```python
from build123d import *

# Parameters (mm, degrees)
ESQUISSE3_R             = 1.5
ESQUISSE3_R_2           = 2
ENL_V_MAT_EXTRU_2_DEPTH = 146.729200917
CHANFREIN1_SIZE         = 0.5


with BuildPart() as part:
    # Esquisse1 → Base-Révolution (revolve)
    with BuildSketch(Plane.XY, mode=Mode.PRIVATE) as base_r_volution_sk:
        with BuildLine():
            Line((0, 0), (0, 4))
            Line((0, 4), (-25, 4))
            ThreePointArc((-25, 4), (-25.936491673, 3.627016654), (-26.936491673, 3.5))
            Line((-26.936491673, 3.5), (-118.063508327, 3.5))
            ThreePointArc((-118.063508327, 3.5), (-119.063508327, 3.627016654), (-120, 4))
            Line((-120, 4), (-145, 4))
            Line((-145, 4), (-145, 0))
            Line((-145, 0), (0, 0))
        make_face()
    revolve(base_r_volution_sk.sketch.rotate(Axis((36, 0, 0), (-1, 0, 0)), 90), axis=Axis((36, 0, 0), (-1, 0, 0)))

    # Esquisse3 → Enlèv. mat.-Extru.2 (cut, through all)
    with BuildSketch(Plane(origin=(0, 10, 0), x_dir=(-1, 0, 0), z_dir=(0, 1, 0))):
        with Locations(Location((5.5, 0, 0), (0, 0, 90))):
            Circle(ESQUISSE3_R)
        with Locations(Location((139.5, 0, 0), (0, 0, 90))):
            Circle(ESQUISSE3_R_2)
    extrude(amount=-ENL_V_MAT_EXTRU_2_DEPTH, mode=Mode.SUBTRACT)

    # Chanfrein1
    chanfrein1_edges = [part.edges().sort_by_distance(p)[0] for p in [
        (0, 0, 4),
        (-145, 0, 4),
    ]]
    chamfer(chanfrein1_edges, length=CHANFREIN1_SIZE)


solid = part.part
```
Verification items for the finished model (mm, model axes). A direction names the side the tool comes from. Coordinates: 2 decimals unless noted, no trailing zeros. Loops run counter-clockwise (first coordinate to the right, second up) from the corner with the lowest first, then second, coordinate; pieces in that order, holes last. Notation, with made-up numbers: (29, 50.25) - (79, 50.25) arc R32 ccw to (79, 87.25) - close; hole circle Ø4 at (-36.5, 70). An arc over 180 degrees is marked (long way). Answer as a JSON object with one key per item and string values.
(1) Cross-section at C-C, the plane x = -139.5. Record the boundary of the cut face in (y, z), then the cut area to 3 significant figures.
Response:
{"outline": "(-3.46, -2) arc R4 ccw to (3.46, -2) - close; (-3.46, 2) - (3.46, 2) arc R4 ccw to start", "area": "19.7 mm²"}
(2) Scan lines: line 1 along X through (y, z) = (-0.75, 0); line 2 along Z through (x, y) = (-139.5, -0.25); line 3 along Y through (x, z) = (-25, 0.25). Record each from-to range of solid material in increasing order.
Response:
{"line 1": "x = -145 to -141.5, -137.5 to -7, -4 to 0", "line 2": "z = -3.99 to -2, 2 to 3.99", "line 3": "y = -3.99 to 3.99"}
(3) Cross-section at D-D, the plane x = -5.5. Record the boundary of the cut face in (y, z), then the cut area to 3 significant figures.
Response:
{"outline": "(-3.71, -1.5) arc R4 ccw to (3.71, -1.5) - close; (-3.71, 1.5) - (3.71, 1.5) arc R4 ccw to start", "area": "26.8 mm²"}
(4) Access from +Z, -Z, +X, -X, +Y, -Y to the whole of each face (thin tool, end or side, straight path). Record for faces 4 (the cylindrical face through (-12.922, 1.532, -3.695)), 5 (the cylindrical face through (-73.138, 3.105, -1.615)).
Response:
{"face 4": "+X, -X", "face 5": "none"}
(5) Cross-section at A-A, the plane y = 0. Record the boundary of the cut face in (x, z), then the cut area to 3 significant figures.
Response:
{"outline": "(-145, -3.5) - (-144.5, -4) - (-120, -4) arc R4 cw to (-118.06, -3.5) - (-26.94, -3.5) arc R4 cw to (-25, -4) - (-0.5, -4) - (0, -3.5) - (0, 3.5) - (-0.5, 4) - (-25, 4) arc R4 cw to (-26.94, 3.5) - (-118.06, 3.5) arc R4 cw to (-120, 4) - (-144.5, 4) - (-145, 3.5) - close; hole circle Ø4 at (-139.5, 0); hole circle Ø3 at (-5.5, 0)", "area": "1,050 mm²"}
(6) Cross-section at B-B, the plane x = -79. Record the boundary of the cut face in (y, z), then the cut area to 3 significant figures.
Response:
{"outline": "circle Ø7 at (0, 0)", "area": "38.5 mm²"}
(7) Go/stop test with flat-tipped pins: pin 1 Ø1.5 at (x, y) = (-23, -2.5) entering from +Z; pin 2 Ø1.5 at (x, z) = (-91, -3) entering from -Y. Record where each tip stops, or that it passes through.
Response:
{"pin 1": "stops at z = 3.6", "pin 2": "stops at y = -2.68"}
(8) Mould release check, pull along X, two halves, no side actions. Record for faces 1 (the flat face through (0, 0, 0)), 2 (the flat face through (-145, 0, 0)), 3 (the cylindrical face through (-140.266, 0.056, 1.847)): pulls with the +X half, pulls with the -X half, needs draft (parallel to the pull), parting line crosses it, or undercut.
Response:
{"face 1": "pulls with the +X half", "face 2": "pulls with the -X half", "face 3": "undercut"}
